```python
from build123d import *

# Parameters (mm, degrees)
SKETCH1_R           = 2.25
BOSS_EXTRUDE1_DEPTH = 5
SKETCH2_R           = 3
BOSS_EXTRUDE2_DEPTH = 1.5
CHAMFER1_SIZE       = 0.4
CHAMFER1_SIZE2      = 0.230940108
FILLET1_R           = 0.1
SKETCH3_R           = 2.1
BOSS_EXTRUDE3_DEPTH = 4.8
CHAMFER2_SIZE       = 0.5
FILLET2_R           = 0.1
SKETCH4_R           = 1.6
BOSS_EXTRUDE4_DEPTH = 6
SKETCH5_R           = 2
BOSS_EXTRUDE5_DEPTH = 0.8
CHAMFER3_SIZE       = 0.5
CHAMFER3_SIZE2      = 0.243866294
CUT_EXTRUDE3_START  = -11.629289
SKETCH6_R           = 1.706133706
CUT_EXTRUDE3_DEPTH  = 11.629289
SKETCH7_W           = 0.634931808
SKETCH7_H           = 0.6
BOSS_EXTRUDE6_DEPTH = 11.329289
CIRPATTERN2_COUNT   = 6
FILLET3_R           = 0.1
FILLET4_R           = 0.1
CUT_EXTRUDE4_REACH  = 20.1
SKETCH8_R           = 1.2446


with BuildPart() as part:
    # Sketch1 → Boss-Extrude1 (new body)
    with BuildSketch(Plane(origin=(0, 0, 0), x_dir=(1, 0, 0), z_dir=(0, 1, 0))):
        with Locations(Location((0, 0, 0), (0, 0, 270))):  # turned: the seam where the file's is
            Circle(SKETCH1_R)
    extrude(amount=BOSS_EXTRUDE1_DEPTH)

    # Sketch2 → Boss-Extrude2 (add)
    with BuildSketch(Plane(origin=(0, 0, 0), x_dir=(-1, 0, 0), z_dir=(0, -1, 0))):
        with Locations(Location((0, 0, 0), (0, 0, 90))):  # turned: the seam where the file's is
            Circle(SKETCH2_R)
    extrude(amount=BOSS_EXTRUDE2_DEPTH)

    # Chamfer1
    chamfer1_edges = [part.edges().sort_by_distance(p)[0] for p in [
        (0, -1.5, 3),
    ]]
    chamfer1_side = [part.faces().sort_by_distance(p)[0] for p in [
        (0, -0.75, 3),
    ]]
    chamfer(chamfer1_edges, length=CHAMFER1_SIZE, length2=CHAMFER1_SIZE2, reference=chamfer1_side[0])

    # Fillet1
    fillet1_edges = [part.edges().sort_by_distance(p)[0] for p in [
        (0, -1.1, 3),
        (0, -1.5, 2.769059892),
    ]]
    fillet(fillet1_edges, radius=FILLET1_R)

    # Sketch3 → Boss-Extrude3 (add)
    with BuildSketch(Plane(origin=(0, -1.5, 0), x_dir=(-1, 0, 0), z_dir=(0, -1, 0))):
        with Locations(Location((0, 0, 0), (0, 0, 90))):  # turned: the seam where the file's is
            Circle(SKETCH3_R)
    extrude(amount=BOSS_EXTRUDE3_DEPTH)

    # Chamfer2
    chamfer2_edges = [part.edges().sort_by_distance(p)[0] for p in [
        (0, -6.3, 2.1),
    ]]
    chamfer(chamfer2_edges, length=CHAMFER2_SIZE)

    # Fillet2
    fillet2_edges = [part.edges().sort_by_distance(p)[0] for p in [
        (0, -6.3, 1.6),
        (0, -5.8, 2.1),
    ]]
    fillet(fillet2_edges, radius=FILLET2_R)

    # Sketch4 → Boss-Extrude4 (add)
    with BuildSketch(Plane(origin=(0, -6.3, 0), x_dir=(-1, 0, 0), z_dir=(0, -1, 0))):
        with Locations(Location((0, 0, 0), (0, 0, 90))):  # turned: the seam where the file's is
            Circle(SKETCH4_R)
    extrude(amount=BOSS_EXTRUDE4_DEPTH)

    # Sketch5 → Boss-Extrude5 (add)
    with BuildSketch(Plane(origin=(0, 5, 0), x_dir=(1, 0, 0), z_dir=(0, 1, 0))):
        with Locations(Location((0, 0, 0), (0, 0, 270))):  # turned: the seam where the file's is
            Circle(SKETCH5_R)
    extrude(amount=BOSS_EXTRUDE5_DEPTH)

    # Chamfer3
    chamfer3_edges = [part.edges().sort_by_distance(p)[0] for p in [
        (0, 5, -2.25),
    ]]
    chamfer3_side = [part.faces().sort_by_distance(p)[0] for p in [
        (0, 2.5, -2.25),
    ]]
    chamfer(chamfer3_edges, length=CHAMFER3_SIZE, length2=CHAMFER3_SIZE2, reference=chamfer3_side[0])

    # Sketch6 → Cut-Extrude3 (cut)
    with BuildSketch(Plane(origin=(0, 5.8, 0), x_dir=(1, 0, 0), z_dir=(0, 1, 0)).offset(CUT_EXTRUDE3_START)):
        with Locations(Location((0, 0, 0), (0, 0, 270))):  # turned: the seam where the file's is
            Circle(SKETCH6_R)
    extrude(amount=CUT_EXTRUDE3_DEPTH, mode=Mode.SUBTRACT)

    # Sketch7 → Boss-Extrude6 (add)
    with BuildSketch(Plane(origin=(0, 5.8, 0), x_dir=(1, 0, 0), z_dir=(0, 1, 0))):
        with Locations((-1.52359961, 0)):
            Rectangle(SKETCH7_W, SKETCH7_H)
    boss_extrude6 = extrude(amount=-BOSS_EXTRUDE6_DEPTH)

    # CirPattern2: Boss-Extrude6 ×6 about axis
    cirpattern2_axis = Axis((0, 0, 0), (0, 1, 0))
    for i in range(1, CIRPATTERN2_COUNT):
        add(boss_extrude6.rotate(cirpattern2_axis, i * 360 / CIRPATTERN2_COUNT))

    # Fillet3
    fillet3_edges = [part.edges().sort_by_distance(p)[0] for p in [
        (-1.206133706, 0.1353555, 0.3),
        (-1.442842451, 5.8, -0.3),
        (-1.442842451, 5.8, 0.3),
        (-1.206133706, 5.8, 0),
        (-1.206133706, 0.1353555, -0.3),
    ]]
    fillet(fillet3_edges, radius=FILLET3_R)

    # Fillet4
    fillet4_edges = [part.edges().sort_by_distance(p)[0] for p in [
        (1.206133706, 0.1353555, -0.3),
        (1.442842451, 5.8, 0.3),
        (1.442842451, 5.8, -0.3),
        (1.206133706, 5.8, 0),
        (1.206133706, 0.1353555, 0.3),
        (0.343259232, 0.1353555, -1.19454243),
        (0.981228847, 5.8, -1.099538216),
        (0.461613604, 5.8, -1.399538216),
        (0.603066853, 5.8, -1.04454243),
        (0.862874474, 0.1353555, -0.89454243),
        (-0.862874474, 0.1353555, -0.89454243),
        (-0.461613604, 5.8, -1.399538216),
        (-0.981228847, 5.8, -1.099538216),
        (-0.603066853, 5.8, -1.04454243),
        (-0.343259232, 0.1353555, -1.19454243),
        (-0.343259232, 0.1353555, 1.19454243),
        (-0.981228847, 5.8, 1.099538216),
        (-0.461613604, 5.8, 1.399538216),
        (-0.603066853, 5.8, 1.04454243),
        (-0.862874474, 0.1353555, 0.89454243),
        (0.862874474, 0.1353555, 0.89454243),
        (0.461613604, 5.8, 1.399538216),
        (0.981228847, 5.8, 1.099538216),
        (0.603066853, 5.8, 1.04454243),
        (0.343259232, 0.1353555, 1.19454243),
    ]]
    fillet(fillet4_edges, radius=FILLET4_R)

    # Sketch8 → Cut-Extrude4 (cut, up to next)
    with BuildSketch(Plane(origin=(0, -12.3, 0), x_dir=(-1, 0, 0), z_dir=(0, -1, 0)), mode=Mode.PRIVATE) as cut_extrude4_sk1:
        with Locations(Location((0, 0, 0), (0, 0, 90))):  # turned: the seam where the file's is
            Circle(SKETCH8_R)
    cut_extrude4_tool1 = extrude(cut_extrude4_sk1.sketch, amount=-CUT_EXTRUDE4_REACH, mode=Mode.PRIVATE) & part.part
    add(cut_extrude4_tool1.solids().sort_by_distance((0, -12.3, 0))[0], mode=Mode.SUBTRACT)


solid = part.part
```
Input: part model. Units: mm. Frame: model coordinates. A direction names the side the tool comes from. Round coordinates to 2 decimals unless told otherwise and drop trailing zeros.
1) Set-up query: faces 1 (the cylindrical face through (0.631, -3.599, -2.003)), 2 (the cylindrical face through (0.9, -0.53, -2.86)), 3 (the cylindrical face through (-1.952, 5.394, -0.434)). Return all of +Z, -Z, +X, -X, +Y, -Y with unobstructed straight access to the full face (end or side cutting, diameter ignored); none if empty.
Ans:
face 1: -Y
face 2: +Y, -Y
face 3: +Y
2) Pull-direction query (Z, two-part tool) for faces 4 (the flat face through (-1, -12.3, -1)), 5 (the flat face through (-1, -5.829, -1)), 6 (the cylindrical face through (-0.97, -9.26, 1.27)); classes: released by +Z, released by -Z, zero draft, split by the parting line, or undercut.
Ans:
face 4: zero draft
face 5: undercut
face 6: split by the parting line
3) Material intervals for line 1 (X direction, y = 2.25, z = 0); line 2 (Z direction, x = -1.5, y = 1.75); line 3 (Z direction, x = -0.5, y = -2.5), sorted ascending.
Ans:
line 1: x = -2.25 to -1.21, 1.21 to 2.25
line 2: z = -1.68 to -0.81, -0.3 to 0.3, 0.81 to 1.68
line 3: z = -2.04 to -1.63, -1.47 to -1.1, 1.1 to 1.47, 1.63 to 2.04
4) Pin query (flat end, axial travel): pin 1 (2 mm diameter, centred on x = 1, y = -3.5, fed in from +Z); pin 2 (1.5 mm diameter, centred on x = 0, z = 0, fed in from +Y); pin 3 (1.5 mm diameter, centred on y = -2, z = -2, fed in from +X); pin 4 (3 mm diameter, centred on x = 0.5, y = -4, fed in from -Z). Return the tip coordinate at first contact, or that it passes through.
Ans:
pin 1: stops at z = 2.1
pin 2: passes through
pin 3: stops at x = 2.37
pin 4: stops at z = -2.1
